Could you check a few things on this drawing? It's one solid part, dimensions in mm from its lowest x, y, z. A direction names the side the tool comes from. Coordinates: 2 decimals unless noted, no trailing zeros. Loops run counter-clockwise (first coordinate to the right, second up) from the corner with the lowest first, then second, coordinate; pieces in that order, holes last. Notation, with made-up numbers: (42, 20.25) -> (100, 20.25) arc R17 ccw to (100, 41.25) -> close; hole circle Ø4 at (-21, -30.75). An arc over 180 degrees is marked (long way). One line per question, with ' | ' between items.
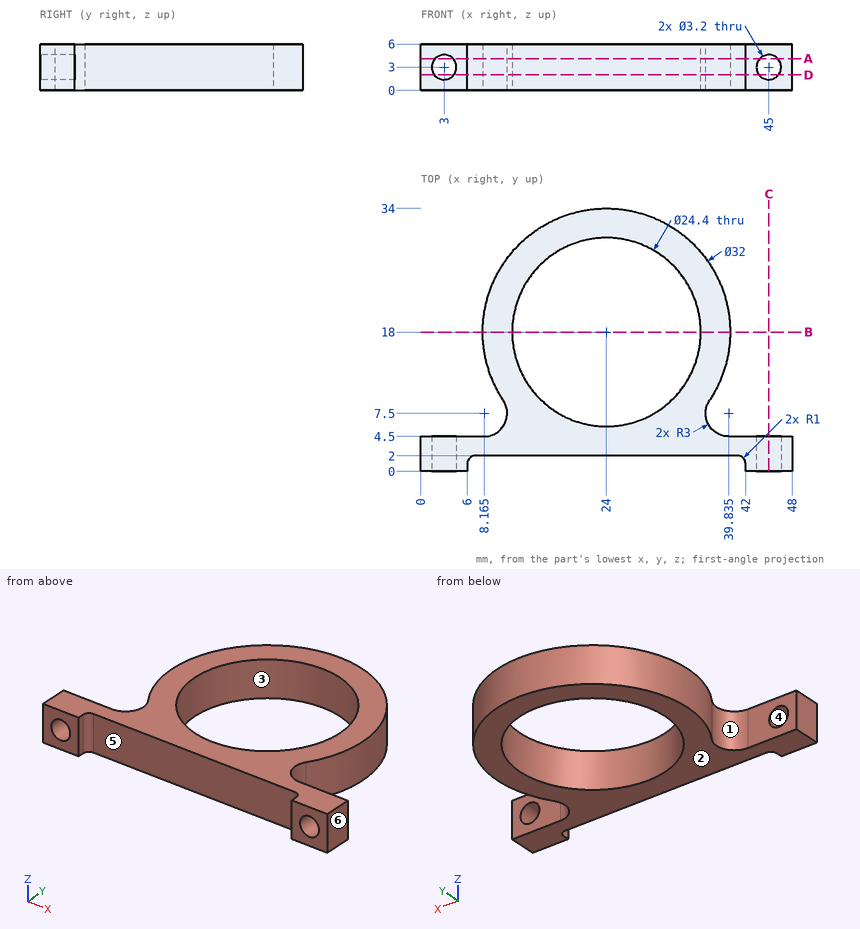
1) If we section it at D-D on z = 2: Please give me the cut outline in (x, y) (3 decimals), and give its area (3 significant figures).
Data:
outline: (0, 0) -> (1.751, 0) -> (1.751, 4.5) -> (0, 4.5) -> close; (4.249, 0) -> (6, 0) -> (6, 1) arc R1 cw to (7, 2) -> (41, 2) arc R1 cw to (42, 1) -> (42, 0) -> (43.751, 0) -> (43.751, 4.5) -> (39.835, 4.5) arc R3 cw to (37.335, 9.158) arc R16 ccw (long way) to (10.665, 9.158) arc R3 cw to (8.165, 4.5) -> (4.249, 4.5) -> close; (46.249, 0) -> (48, 0) -> (48, 4.5) -> (46.249, 4.5) -> close; hole circle Ø24.4 at (24, 18) | area: 448 mm²
2) If we section it at A-A on z = 4.1: Please give me the cut outline in (x, y) (3 decimals).
Data:
outline: (0, 0) -> (1.838, 0) -> (1.838, 4.5) -> (0, 4.5) -> close; (4.162, 0) -> (6, 0) -> (6, 1) arc R1 cw to (7, 2) -> (41, 2) arc R1 cw to (42, 1) -> (42, 0) -> (43.838, 0) -> (43.838, 4.5) -> (39.835, 4.5) arc R3 cw to (37.335, 9.158) arc R16 ccw (long way) to (10.665, 9.158) arc R3 cw to (8.165, 4.5) -> (4.162, 4.5) -> close; (46.162, 0) -> (48, 0) -> (48, 4.5) -> (46.162, 4.5) -> close; hole circle Ø24.4 at (24, 18)
3) If we section it at C-C on x = 45: Please give me the cut outline in (y, z).
Data:
outline: (0, 0) -> (4.5, 0) -> (4.5, 1.4) -> (0, 1.4) -> close; (0, 4.6) -> (4.5, 4.6) -> (4.5, 6) -> (0, 6) -> close
4) I'm going to push flat-ended pins straight in: pin 1 Ø1.8 at (x, z) = (45, 4) entering from +Y; pin 2 Ø1.8 at (x, z) = (31.5, 3) entering from -Y. Where does each tip first touch, or does it pass through?
Data:
pin 1: y = 4.5 | pin 2: y = 2
5) If we section it at B-B on y = 18: Please give me the cut outline in (x, z).
Data:
outline: (8, 0) -> (11.8, 0) -> (11.8, 6) -> (8, 6) -> close; (36.2, 0) -> (40, 0) -> (40, 6) -> (36.2, 6) -> close
6) On a 3-axis mill with a long thin cutter (end or side, diameter ignored), from which of +Z, -Z, +X, -X, +Y, -Y can I reach the whole of each face in a straight line? I mean the marked faces 5 and 6. Say none if no direction works.
Data:
face 5: +Z, -Z, -Y | face 6: +Z, -Z, +X, +Y, -Y
7) We'd pull the mould along X, two halves only. Please class the marked faces 1, 2, 3 and 4: pulls with the +X half, pulls with the -X half, needs draft (parallel to the pull), parting line crosses it, or undercut.
Data:
face 1: pulls with the -X half | face 2: needs draft | face 3: undercut | face 4: undercut
8) I need wall thicknesses on line 1 along Z through (x, y) = (3, 2.6); line 2 along Y through (x, z) = (24, 1.3); line 3 along X through (y, z) = (23.5, 5.45) (3 decimals). Which ranges of each line are inside material? Lowest first, please. Write a range as from..to.
Data:
line 1: 0..1.4, 4.6..6 | line 2: 2..5.8, 30.2..34 | line 3: 8.975..13.11, 34.89..39.025
